Part print with two shaded views. Sizes in mm from the minimum x, y, z corner. A direction names the side the tool comes from. Give positions to 0.01 mm unless a question says otherwise; leave off trailing zeros. Write each loop counter-clockwise with the first axis right and the second up, starting at its lowest first coordinate (ties: lowest second). Pieces come first, ordered by that corner, then holes. Notation, with made-up numbers: (30.5, 12) -> (76.5, 12) arc R17 cw to (76.5, 38) -> close; hole circle Ø9 at (58.5, -33). An arc over 180 degrees is marked (long way). Answer as a JSON object with one key per item and string values.
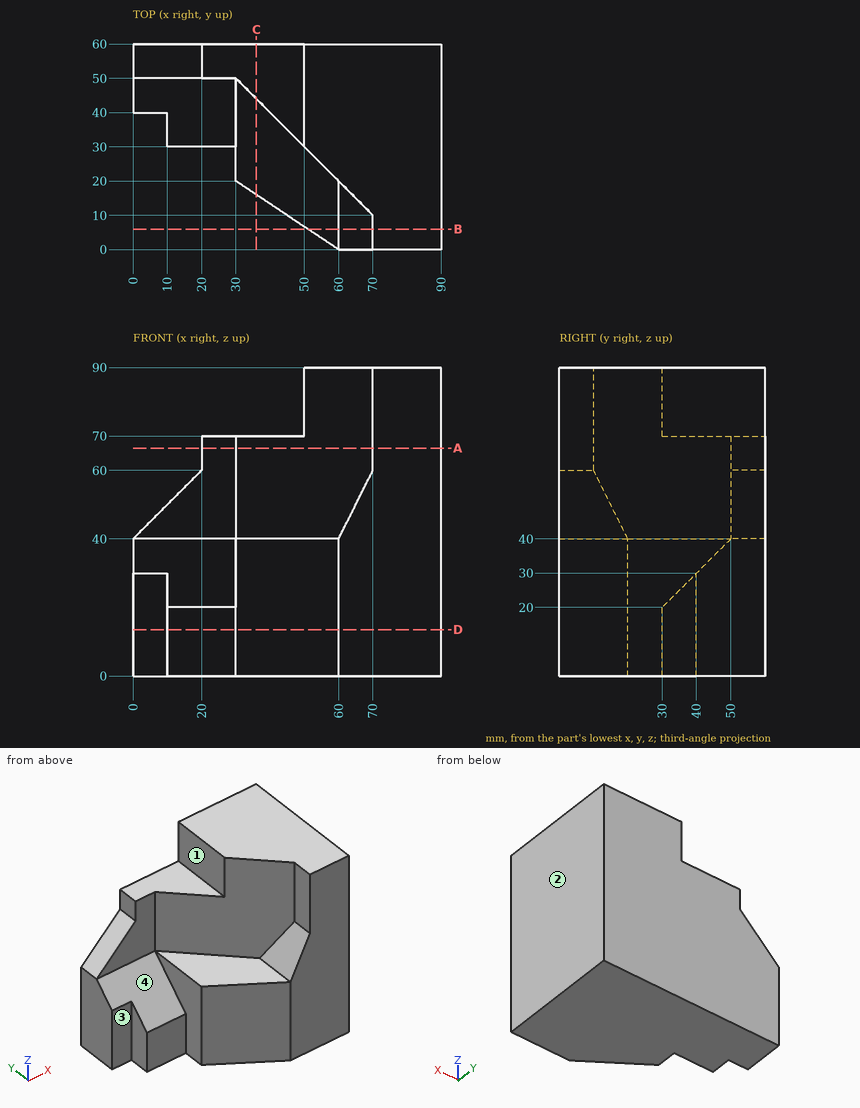
1) Wall check: probe 1 along X at (y, z) = (23, 35.5); probe 2 along X at (y, z) = (54, 72); probe 3 along Z at (x, y) = (55, 4.5). Give the ranges that are in metal, low to high.
Model answer:
{"probe 1": "x = 30 to 90", "probe 2": "x = 50 to 90", "probe 3": "z = 0 to 40"}
2) 3-axis set-ups, long thin cutter, end or side, ignore diameter. For the marked faces 1, 2, 3 and 4: which of +Z, -Z, +X, -X, +Y, -Y reach the whole face in a straight line?
Model answer:
{"face 1": "+Z, -X, +Y, -Y", "face 2": "+Z, -Z, +X, +Y, -Y", "face 3": "+Z, -Z, -X, -Y", "face 4": "+Z, -X, -Y"}
3) Slice it at D-D (z = 13.5). List the corners of the cut face in (x, y), then the cut area to 3 significant figures.
Model answer:
{"outline": "(0, 40) -> (10, 40) -> (10, 30) -> (30, 30) -> (30, 20) -> (60, 0) -> (90, 0) -> (90, 60) -> (0, 60) -> close", "area": "4,100 mm2"}
4) Slice it at A-A (z = 66.5). List the corners of the cut face in (x, y), then the cut area to 3 significant figures.
Model answer:
{"outline": "(20, 50) -> (30, 50) -> (70, 10) -> (70, 0) -> (90, 0) -> (90, 60) -> (20, 60) -> close", "area": "2,500 mm2"}
5) Slice it at B-B (y = 6). List the corners of the cut face in (x, z).
Model answer:
{"outline": "(51, 0) -> (90, 0) -> (90, 90) -> (70, 90) -> (70, 60) -> (60, 40) -> (51, 40) -> close"}
6) Slice it at C-C (x = 36). List the corners of the cut face in (y, z).
Model answer:
{"outline": "(16, 0) -> (60, 0) -> (60, 70) -> (44, 70) -> (44, 40) -> (16, 40) -> close"}
7) Pin check, flat tips, straight feed: pin 1 (3 mm diameter, centred on y = 34.5, z = 21.5, fed in from -X); pin 2 (1.5 mm diameter, centred on x = 53, z = 59.5, fed in from -Y); pin 3 (22 mm diameter, centred on y = 38, z = 75, fed in from -X). Stop position of each tip, or through.
Model answer:
{"pin 1": "stops at x = 10", "pin 2": "stops at y = 26.25", "pin 3": "stops at x = 32.2"}
